The listing builds one solid part. Answer for the finished solid, in the listing's coordinates (mm). A direction names the side the tool comes from. Round coordinates to 2 decimals unless told otherwise and drop trailing zeros. Loops run counter-clockwise (first coordinate to the right, second up) from the corner with the lowest first, then second, coordinate; pieces in that order, holes last. Notation, with made-up numbers: (-5, 83) - (53, 83) arc R16 cw to (53, 103) - close; hole circle Ø1 at (10, 83.5). An arc over 180 degrees is marked (long way). One line per question, with ' | ' between items. Start each with the question number.
from build123d import *

# Parameters (mm, degrees)
SKETCH1_W           = 12.7
SKETCH1_H           = 139.7
BOSS_EXTRUDE1_DEPTH = 12.7
SKETCH2_W           = 63.5
SKETCH2_H           = 12.7
BOSS_EXTRUDE2_DEPTH = 12.7
SKETCH3_W           = 12.7
SKETCH3_H           = 88.9
BOSS_EXTRUDE3_DEPTH = 12.7
BOSS_EXTRUDE5_DEPTH = 12.7
BOSS_EXTRUDE6_START = -19.05
BOSS_EXTRUDE6_DEPTH = 12.7
SKETCH6_R           = 1.778
CUT_EXTRUDE1_DEPTH  = 89.9


with BuildPart() as part:
    # Sketch1 → Boss-Extrude1 (new body)
    with BuildSketch(Plane.XY):
        with Locations((6.35, 69.85)):
            Rectangle(SKETCH1_W, SKETCH1_H)
    extrude(amount=BOSS_EXTRUDE1_DEPTH)

    # Sketch2 → Boss-Extrude2 (add)
    with BuildSketch(Plane.ZY):
        with Locations((-31.75, 6.35)):
            Rectangle(SKETCH2_W, SKETCH2_H)
    extrude(amount=-BOSS_EXTRUDE2_DEPTH)

    # Sketch3 → Boss-Extrude3 (add)
    with BuildSketch(Plane.ZY):
        with Locations((-69.85, 44.45)):
            Rectangle(SKETCH3_W, SKETCH3_H)
    extrude(amount=-BOSS_EXTRUDE3_DEPTH)

    # Sketch4 → Boss-Extrude5 (add)
    with BuildSketch(Plane.XY.offset(12.7)):
        Polygon((12.7, 0), (39.453062828, -27.127175108), (26.753062828, -27.127175108), (0, 0), align=None)
    extrude(amount=-BOSS_EXTRUDE5_DEPTH)

    # Sketch5 → Boss-Extrude6 (add)
    with BuildSketch(Plane(origin=(0, 0, -76.2), x_dir=(-1, 0, 0), z_dir=(0, 0, -1)).offset(BOSS_EXTRUDE6_START)):
        Polygon((0, 0), (-26.753062828, -27.127175108), (-39.453062828, -27.127175108), (-12.7, 0), align=None)
    extrude(amount=-BOSS_EXTRUDE6_DEPTH)

    # Sketch6 → Cut-Extrude1 (cut, through all)
    with BuildSketch(Plane.XY.offset(12.7)):
        with BuildLine():
            ThreePointArc((6.35, 131.572), (8.128, 133.35), (6.35, 135.128))
            Line((6.35, 135.128), (6.35, 131.572))
        make_face()
        with Locations((6.35, 112.7125)):
            Circle(SKETCH6_R)
        with Locations((6.35, 123.03125)):
            Circle(SKETCH6_R)
    extrude(amount=-CUT_EXTRUDE1_DEPTH, mode=Mode.SUBTRACT)


solid = part.part
(1) Find section B-B on z = -54.5. Write down the section's boundary in (x, y).
(2) Find section C-C on y = -15.5. Write down the section's boundary in (x, z), plus the area to 3 significant figures.
(3) Each of these flat-tipped pins is pushed along its axis until it touches: P1, Ø6.5, axis at x = 5, z = -70.5, coming from the -Y side; P2, Ø3, axis at y = 133, z = 5, coming from the +X side; P3, Ø4.5, axis at x = 6.35, y = 123.03, coming from the +Z side; P4, Ø4, axis at x = 4.5, z = -44.5, coming from the +Y side. Where does it stop, or does it pass through?
(4) Determine the mould class of faces 5 (the flat face through (6, 50, -63.5)), 6 (the flat face through (6, 0, -67)) for opening direction Z: pulls with the +Z half, pulls with the -Z half, needs draft (parallel to the pull), parting line crosses it, or undercut.
(5) Find section D-D on z = -18. Write down the section's boundary in (x, y), plus the area to 3 significant figures.
(6) A tool of negligible diameter and unlimited length cuts with its end or side. For faces 1 (the flat face through (20, -14, 0)), 2 (the flat face through (6, 88.9, -70)), 3 (the flat face through (6, 77, 0)), 4 (the flat face through (6.35, 133, 6)), from which of +Z, -Z, +X, -X, +Y, -Y can it reach the whole face along a straight path? Write none if from no direction.
(7) Find section A-A on y = 133.35. Write down the section's boundary in (x, z).
(8) Consider L1, parallel to Z at x = 5, y = 49.5; L2, parallel to Y at x = 6, z = 9; L3, parallel to X at y = 133, z = 1. Determine where each line is inside the solid, lowest interval first.
Answer below:
1) outline: (0, 0) - (26.75, -27.13) - (39.45, -27.13) - (12.7, 0) - (12.7, 12.7) - (0, 12.7) - close
2) outline: (15.29, -57.15) - (27.99, -57.15) - (27.99, -44.45) - (15.29, -44.45) - close; (15.29, 0) - (27.99, 0) - (27.99, 12.7) - (15.29, 12.7) - close | area: 323 mm2
3) P1: y = 0 | P2: x = 12.7 | P3: z = 12.7 | P4: y = 12.7
4) face 5: undercut | face 6: needs draft
5) outline: (0, 0) - (12.7, 0) - (12.7, 12.7) - (0, 12.7) - close | area: 161 mm2
6) face 1: +X, -X, -Y | face 2: -Z, +X, -X, +Y | face 3: +X, -X, +Y | face 4: +Z, -Z
7) outline: (0, 0) - (6.35, 0) - (6.35, 12.7) - (0, 12.7) - close; (8.13, 0) - (12.7, 0) - (12.7, 12.7) - (8.13, 12.7) - close
8) L1: -76.2 to -63.5, 0 to 12.7 | L2: -6.08 to 110.97, 114.46 to 121.29, 124.77 to 139.7 | L3: 0 to 6.35, 8.09 to 12.7
